Part model, mm, in its own coordinate system. A direction names the side the tool comes from. Coordinates: 2 decimals unless noted, no trailing zeros. Write each loop counter-clockwise with the first axis right and the second up, starting at its lowest first coordinate (ties: lowest second). Pieces come first, ordered by that corner, then holes. Notation, with made-up numbers: M 5.25,-2 L 62.25,-2 A20 cw 62.25,16 Z; hole C 23,-11 d11. An arc over 180 degrees is marked long. Use a Markdown table: item, result. Add a question column.
Q1. Tool access for faces 1 (the flat face through (7.938, 2, 4)), 2 (the flat face through (9.525, 0, 4)): list every direction of +Z, -Z, +X, -X, +Y, -Y with a clear straight run to the whole face (end or side of a thin tool).
Q2. Slice it at B-B on y = 2.5. Write the cut outline in (x, z) (1 decimal), then the cut area to 3 significant figures.
Q3. Slice it at A-A on z = -140.5. Write the cut outline in (x, y) (1 decimal), then the cut area to 3 significant figures.
Q4. Pin check, flat tips, straight feed: pin 1 Ø8 at (x, z) = (3.175, 215.9) entering from +Y; pin 2 Ø1 at (x, z) = (2.5, -65) entering from +Y; pin 3 Ø3 at (x, z) = (3.175, -241.3) entering from -Y; pin 4 Ø1 at (y, z) = (5.5, -189.5) entering from -X. Stop position of each tip, or through.
Q5. Wall check: L1, parallel to X at y = -8.35, z = -215.9 (3 decimals); L2, parallel to X at y = -8.55, z = -215.9 (3 decimals); L3, parallel to Y at x = -3.5, z = 55.5 (1 decimal). Give the ranges that are in metal, low to high. Write a range as from..to.
from build123d import *

# Parameters (mm, degrees)
BOSS_EXTRUDE1_DEPTH        = 254
F_10_CLEARANCE_HOLE1_D     = 4.9784
F_10_CLEARANCE_HOLE1_DEPTH = 3.302
F_10_CLEARANCE_HOLE1_TIP   = 1.495662253


with BuildPart() as part:
    # Sketch2 → Boss-Extrude1 (new, symmetric)
    with BuildSketch(Plane.XY):
        with BuildLine():
            Line((-9.525, -9.525), (9.525, -9.525))
            Line((9.525, -9.525), (9.525, 9.525))
            Line((9.525, 9.525), (8.73125, 9.525))
            ThreePointArc((8.73125, 9.525), (8.169983992, 9.292516008), (7.9375, 8.73125))
            Line((7.9375, 8.73125), (7.9375, -5.5499))
            ThreePointArc((7.9375, -5.5499), (7.238188151, -7.238188151), (5.5499, -7.9375))
            Line((5.5499, -7.9375), (-8.73125, -7.9375))
            ThreePointArc((-8.73125, -7.9375), (-9.292516008, -8.169983992), (-9.525, -8.73125))
            Line((-9.525, -8.73125), (-9.525, -9.525))
        make_face()
    extrude(amount=BOSS_EXTRUDE1_DEPTH, both=True)

    # #10 Clearance Hole1
    with Locations(Plane(origin=(0, -9.525, 0), x_dir=(-1, 0, 0), z_dir=(0, -1, 0))):
        with Locations((-3.175, 241.3), (-3.175, 215.9), (-3.175, -241.3), (-3.175, -215.9)):
            Hole(F_10_CLEARANCE_HOLE1_D / 2, depth=F_10_CLEARANCE_HOLE1_DEPTH)
            with Locations((0, 0, -(F_10_CLEARANCE_HOLE1_DEPTH + F_10_CLEARANCE_HOLE1_TIP / 2))):  # 118° drill point
                Cone(0, F_10_CLEARANCE_HOLE1_D / 2, F_10_CLEARANCE_HOLE1_TIP, mode=Mode.SUBTRACT)


solid = part.part
Recorded:
| question | item | result |
|---|---|---|
| 1 | face 1 | +Z, -Z, -X, +Y |
| 1 | face 2 | +Z, -Z, +X, +Y, -Y |
| 2 | outline | M 7.9,-254 L 9.5,-254 L 9.5,254 L 7.9,254 Z |
| 2 | area | 806 mm² |
| 3 | outline | M -9.5,-9.5 L 9.5,-9.5 L 9.5,9.5 L 8.7,9.5 A0.8 ccw 7.9,8.7 L 7.9,-5.5 A2.4 cw 5.5,-7.9 L -8.7,-7.9 A0.8 ccw -9.5,-8.7 Z |
| 3 | area | 58.9 mm² |
| 4 | pin 1 | y = -7.3 |
| 4 | pin 2 | y = -7.94 |
| 4 | pin 3 | through |
| 4 | pin 4 | x = 7.94 |
| 5 | L1 | -9.427..0.686, 5.664..9.525 |
| 5 | L2 | -9.504..0.686, 5.664..9.525 |
| 5 | L3 | -9.5..-7.9 |
